Here's how the part is built. I have some questions about the finished solid (model axes, mm). Face numbers are marked on the shaded views. Give positions to 0.01 mm unless a question says otherwise; leave off trailing zeros. Write each loop counter-clockwise with the first axis right and the second up, starting at its lowest first coordinate (ties: lowest second). Pieces come first, ordered by that corner, then holes. Notation, with made-up numbers: (74.25, -14) -> (125.25, -14) arc R28 ccw to (125.25, 25) -> close; hole circle Ø2 at (5.5, 23). An arc over 180 degrees is marked (long way). Answer as CSV lines item,"result". Start each with the question number.
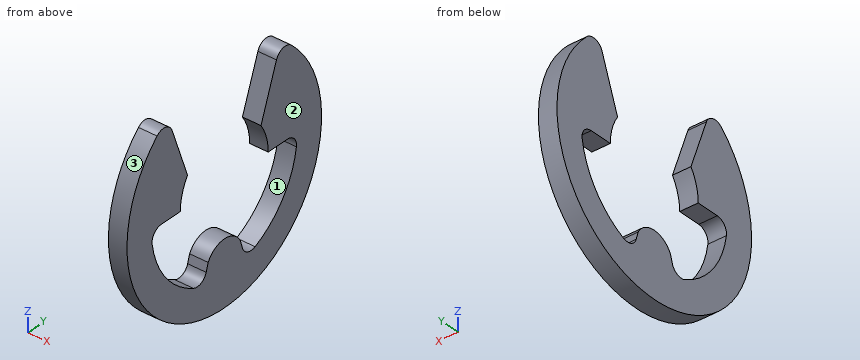
from build123d import *

# Parameters (mm, degrees)
EXTRUDE1_DEPTH          = 0.35
FILLET1_R               = 0.42
CUT_EXTRUDE1_DEPTH      = 7.267675008
CUT_EXTRUDE1_DEPTH_BACK = 7.267675008


with BuildPart() as part:
    # Sketch1 → Extrude1 (new, symmetric)
    with BuildSketch(Plane(origin=(0, 0, 0), x_dir=(0, 0, -1), z_dir=(1, 0, 0))):
        with BuildLine():
            Line((-3.59727207, -2.576869934), (-1.100499886, -1.67))
            ThreePointArc((-1.100499886, -1.67), (-0.574456265, -1.915724406), (0, -2))
            Line((0, -2), (0, -3.316129032))
            ThreePointArc((0, -3.316129032), (1.979664969, -2.660383125), (3.17639466, -0.952485548))
            Line((3.17639466, -0.952485548), (1.915724406, -0.574456265))
            ThreePointArc((1.915724406, -0.574456265), (2, 0), (1.915724406, 0.574456265))
            Line((1.915724406, 0.574456265), (3.17639466, 0.952485548))
            ThreePointArc((3.17639466, 0.952485548), (1.979664969, 2.660383125), (0, 3.316129032))
            Line((0, 3.316129032), (0, 2))
            ThreePointArc((0, 2), (-0.574456265, 1.915724406), (-1.100499886, 1.67))
            Line((-1.100499886, 1.67), (-3.59727207, 2.576869934))
            ThreePointArc((-3.59727207, 2.576869934), (4.425, 0), (-3.59727207, -2.576869934))
        make_face()
    extrude(amount=EXTRUDE1_DEPTH, both=True)

    # Fillet1
    fillet1_edges = [part.edges().sort_by_distance(p)[0] for p in [
        (0, -2.576869934, 3.59727207),
        (0, -3.316129032, 0),
        (0, -0.952485548, -3.17639466),
        (0, 0.952485548, -3.17639466),
        (0, 3.316129032, 0),
        (0, 2.576869934, 3.59727207),
    ]]
    fillet(fillet1_edges, radius=FILLET1_R)

    # Sketch4 → Cut-Extrude1 (cut, two sides)
    with BuildSketch(Plane(origin=(0, 0, 0), x_dir=(0, 0, -1), z_dir=(1, 0, 0))) as cut_extrude1_sk:
        with BuildLine():
            Line((0, 2.865512759), (0, -2.865512759))
            ThreePointArc((0, -2.865512759), (0.145392765, -3.183303361), (0.480908888, -3.281072751))
            ThreePointArc((0.480908888, -3.281072751), (1.979664969, -2.660383125), (3.004685012, -1.403060846))
            ThreePointArc((3.004685012, -1.403060846), (3.007405078, -1.053600513), (2.744766364, -0.823055878))
            ThreePointArc((2.744766364, -0.823055878), (2, 0), (2.744766364, 0.823055878))
            ThreePointArc((2.744766364, 0.823055878), (3.007405078, 1.053600513), (3.004685012, 1.403060846))
            ThreePointArc((3.004685012, 1.403060846), (1.979664969, 2.660383125), (0.480908888, 3.281072751))
            ThreePointArc((0.480908888, 3.281072751), (0.145392765, 3.183303361), (0, 2.865512759))
        make_face()
    extrude(amount=CUT_EXTRUDE1_DEPTH, mode=Mode.SUBTRACT)
    extrude(cut_extrude1_sk.sketch, amount=-CUT_EXTRUDE1_DEPTH_BACK, mode=Mode.SUBTRACT)


solid = part.part
Item 1: If we section it at A-A (z = 2.25): Please give me the cut outline in (x, y), and give its area (3 significant figures).
Item 2: If we section it at B-B (y = -2.75): Please give me the cut outline in (x, z).
Item 3: I'm going to push flat-ended pins straight in: pin 1 (1 mm diameter, centred on y = 1, z = -0.5, fed in from +X); pin 2 (4 mm diameter, centred on y = 3.5, z = -3, fed in from +X). Where does each tip first touch, or does it pass through?
Item 4: If we section it at D-D (y = 0): Please give me the cut outline in (x, z) (3 decimals).
Item 5: We'd pull the mould along Y, two halves only. Please class the marked faces 1, 2 and 3: released by +Y, released by -Y, zero draft, split by the parting line, or undercut.
Item 6: If I drill on line 1 (Y direction, x = -0.2, z = -2.25); line 2 (Y direction, x = -0.2, z = -1.5); line 3 (Y direction, x = -0.25, z = 1.25), over which ranges is the centre line in solid material (lowest first)? Write a range as [from, to].
Final values:
1,outline,"(-0.35, -3.81) -> (0.35, -3.81) -> (0.35, -2.09) -> (-0.35, -2.09) -> close; (-0.35, 2.09) -> (0.35, 2.09) -> (0.35, 3.81) -> (-0.35, 3.81) -> close"
1,area,"2.41 mm2"
2,outline,"(-0.35, -3.47) -> (0.35, -3.47) -> (0.35, -1.85) -> (-0.35, -1.85) -> close; (-0.35, 0) -> (0.35, 0) -> (0.35, 3.31) -> (-0.35, 3.31) -> close"
3,pin 1,"through"
3,pin 2,"x = 0.35"
4,outline,"(-0.35, -4.425) -> (0.35, -4.425) -> (0.35, -2) -> (-0.35, -2) -> close"
5,face 1,"undercut"
5,face 2,"zero draft"
5,face 3,"split by the parting line"
6,line 1,"[-3.81, -2.44], [-0.59, 0.59], [2.44, 3.81]"
6,line 2,"[-4.16, -2.96], [2.96, 4.16]"
6,line 3,"[-4.24, -1.72], [1.72, 4.24]"
